Input: part model. Units: mm. Frame: model coordinates. Coordinates: 2 decimals unless noted, no trailing zeros. Write each loop counter-clockwise with the first axis right and the second up, starting at its lowest first coordinate (ties: lowest second). Pieces come first, ordered by that corner, then holes.
1) Section query B-B (z = -4.75). Output: boundary loops of the cut face in (x, y) (3 decimals).
2) Section query A-A (y = 0). Output: boundary loops of the cut face in (x, z).
3) Section query C-C (x = 24). Output: boundary loops of the cut face in (y, z), then the cut area to 3 significant figures.
4) Draft query along X for faces 1 (the flat face through (19, 114, -6.35)), 2 (the cylindrical face through (12.71, -0.71, -6.26)), 3 (the flat face through (0, 37, -5)), 4 (the cylindrical face through (28.431, 111.293, -3.131)). Return one class per face: pulls with the +X half, pulls with the -X half, needs draft (parallel to the pull), parting line crosses it, or undercut.
5) Line query: L1, parallel to X at y = 0, z = -5.25; L2, parallel to Y at x = 7, z = -5.75; L3, parallel to Y at x = 26.5, z = -4.5. Output: solid intervals per line, ascending.
6) Section query D-D (y = 45). Output: boundary loops of the cut face in (x, z).
Autodesk Inventor part; units mm, degrees
ref_plane "YZ Plane" through (0, 0, 0) normal (1, 0, 0) x (0, 1, 0)
ref_plane "XZ Plane" through (0, 0, 0) normal (0, 1, 0) x (-1, 0, 0)
ref_plane "XY Plane" through (0, 0, 0) normal (0, 0, 1) x (1, 0, 0)
sketch "Sketch1" plane through (0, 0, 0) normal (1, 0, 0) x (0, 1, 0)
  line L0 (0, 0) -> (114.554, 0)
  line L1 (0, 0) -> (-19.05, 0)
  line L2 (-19.05, 0) -> (-19.05, -12.7)
  line L3 (-19.05, -12.7) -> (19.05, -12.7)
  line L4 (101.854, -6.35) -> (114.554, -6.35)
  line L5 (114.554, -6.35) -> (127.254, -6.35)
  line L6 (127.254, -6.35) -> (127.254, 0)
  line L7 (127.254, 0) -> (114.554, 0)
  line L8 (114.554, 0) -> (114.554, -6.35) construction
  line L9 (101.854, 0) -> (101.854, -6.35) construction
  line L10 (19.05, -12.7) -> (101.854, -6.35)
  dimension "d0" = 114.554
  dimension "d1" = 19.05
  dimension "d2" = 12.7
  dimension "d3" = 38.1
  dimension "d4" = 12.7
  dimension "d5" = 25.4
  dimension "d6" = 6.35
extrude "Extrusion1" add sketch "Sketch1" along normal blind 38.1
sketch "Sketch2" plane through (0, -19.05, -12.7) normal (0, 0, -1) x (-1, 0, 0)
  line L0 (0, 38.1) -> (0, 0)
  line L1 (0, 38.1) -> (-38.1, 38.1)
  line L2 (-38.1, 0) -> (-38.1, 38.1)
  line L3 (0, 0) -> (-38.1, 0)
  line L4 (0, 19.05) -> (-38.1, 19.05) construction
  line L5 (-28.575, 38.1) -> (-28.575, 0) construction
  line L6 (-9.525, 38.1) -> (-9.525, 32.2712) construction
  line L7 (-9.525, 32.2712) -> (-9.525, 0) construction
  point P0 (-28.575, 19.05)
  point P1 (-9.525, 19.05)
  dimension "d9" = 9.525
  dimension "d10" = 9.525
sketch "Sketch3" plane through (0, 101.854, -6.35) normal (0, 0, -1) x (-1, 0, 0)
  line L0 (0, 25.4) -> (0, 0)
  line L1 (0, 25.4) -> (-38.1, 25.4)
  line L2 (-38.1, 0) -> (-38.1, 25.4)
  line L3 (0, 0) -> (-38.1, 0)
  line L4 (-38.1, 12.7) -> (0, 12.7) construction
  line L5 (-28.575, 25.4) -> (-28.575, 0) construction
  line L6 (-9.525, 25.4) -> (-9.525, 0) construction
  point P0 (0, -101.854)
  point P1 (-28.575, 12.7)
  point P2 (-9.525, 12.7)
  dimension "d11" = 9.525
  dimension "d12" = 9.525
hole "Hole1" at (9.525, 0, -12.7) at (28.575, 0, -12.7) direction (0, 0, 1) diameter 6.5278 end through all
hole "Hole2" at (28.575, 114.554, -6.35) at (9.525, 114.554, -6.35) direction (0, 0, 1) diameter 6.5278 end through all
fillet_without_effect "Fillet1"
equation "\"d9\" = d10"
equation "\"d12\" = d11"
properties part number "Y_shaft_support_brace_A" material "Aluminum 6061"
Answer:
1. outline: (0, -19.05) - (38.1, -19.05) - (38.1, 127.254) - (0, 127.254) - close; hole circle Ø6.528 at (9.525, 0); hole circle Ø6.528 at (9.525, 114.554); hole circle Ø6.528 at (28.575, 0); hole circle Ø6.528 at (28.575, 114.554)
2. outline: (0, -12.7) - (6.26, -12.7) - (6.26, 0) - (0, 0) - close; (12.79, -12.7) - (25.31, -12.7) - (25.31, 0) - (12.79, 0) - close; (31.84, -12.7) - (38.1, -12.7) - (38.1, 0) - (31.84, 0) - close
3. outline: (-19.05, -12.7) - (19.05, -12.7) - (101.85, -6.35) - (127.25, -6.35) - (127.25, 0) - (-19.05, 0) - close
3. area: 1,430 mm2
4. face 1: needs draft
4. face 2: undercut
4. face 3: pulls with the -X half
4. face 4: undercut
5. L1: x = 0 to 6.26, 12.79 to 25.31, 31.84 to 38.1
5. L2: y = -19.05 to -2.07, 2.07 to 112.49, 116.62 to 127.25
5. L3: y = -19.05 to -2.52, 2.52 to 112.03, 117.07 to 127.25
6. outline: (0, -10.71) - (38.1, -10.71) - (38.1, 0) - (0, 0) - close
